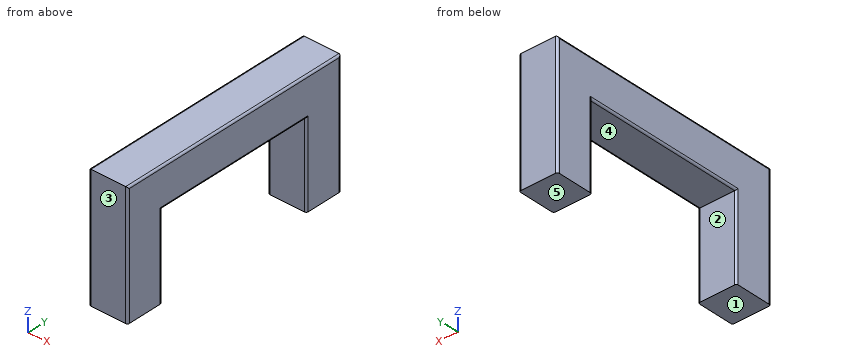
from build123d import *

# Parameters (mm, degrees)
F1_DEPTH = 100
F2_R     = 5


with BuildPart() as f1:
    # F0 (on Right) → F1 (new body)
    with BuildSketch(Plane.YZ):
        Polygon((0, 220), (0, 0), (100, 0), (100, 320), (-520, 320), (-520, 0), (-420, 0), (-420, 220), align=None)
    extrude(amount=F1_DEPTH)

    # F2
    f2_edges = [f1.edges().sort_by_distance(p)[0] for p in [
        (100, -520, 160),
        (100, -420, 110),
        (100, -210, 220),
        (100, 0, 110),
        (100, 100, 160),
        (0, -520, 160),
        (0, 0, 110),
        (0, -210, 220),
        (0, -420, 110),
        (0, 100, 160),
        (0, -210, 320),
        (100, -210, 320),
    ]]
    fillet(f2_edges, radius=F2_R)


solid = f1.part
Input: part model. Units: mm. Frame: model coordinates. Face numbers are marked on the shaded views. A direction names the side the tool comes from. Coordinates: 2 decimals unless noted, no trailing zeros. Write each loop counter-clockwise with the first axis right and the second up, starting at its lowest first coordinate (ties: lowest second). Pieces come first, ordered by that corner, then holes. Notation, with made-up numbers: M -33,58 L -4,58 A26 ccw -4,76 Z; hole C 56.25,-25.5 d6. An arc over 180 degrees is marked long. Answer as a JSON object with one key per item and string values. Group by question number.
(1) Section B-B on x = 18. Output: boundary loops of the cut face in (y, z).
(2) Set-up query: the marked faces 4 and 5. Return all of +Z, -Z, +X, -X, +Y, -Y with unobstructed straight access to the full face (end or side cutting, diameter ignored); none if empty.
(3) Mould query, pull axis Y, two halves, no side actions, for the marked faces 1, 2 and 3. Classes: pulls with the +Y half, pulls with the -Y half, needs draft (parallel to the pull), parting line crosses it, or undercut.
(4) Ray query, line 1 along Y through (x, z) = (91.5, 173.5); line 2 along Z through (x, y) = (73.5, -51). Return the intervals inside material, ascending. Write a range as [from, to].
(5) Section C-C on y = -332. Output: boundary loops of the cut face in (x, z), plus the area to 3 significant figures.
(6) Section A-A on z = 21.5. Output: boundary loops of the cut face in (x, y), plus the area to 3 significant figures.
Result set:
{
 "1": {"outline": "M -520,0 L -420,0 L -420,220 L 0,220 L 0,0 L 100,0 L 100,320 L -520,320 Z"},
 "2": {"face 4": "-Z, +X, -X", "face 5": "-Z, +X, -X, +Y, -Y"},
 "3": {"face 1": "needs draft", "face 2": "undercut", "face 3": "pulls with the -Y half"},
 "4": {"line 1": "y = [-520, -420], [0, 100]", "line 2": "z = [220, 320]"},
 "5": {"outline": "M 0,225 A5 ccw 5,220 L 95,220 A5 ccw 100,225 L 100,315 A5 ccw 95,320 L 5,320 A5 ccw 0,315 Z", "area": "9,980 mm2"},
 "6": {"outline": "M 0,-515 A5 ccw 5,-520 L 95,-520 A5 ccw 100,-515 L 100,-425 A5 ccw 95,-420 L 5,-420 A5 ccw 0,-425 Z; M 0,5 A5 ccw 5,0 L 95,0 A5 ccw 100,5 L 100,95 A5 ccw 95,100 L 5,100 A5 ccw 0,95 Z", "area": "20,000 mm2"}
}
